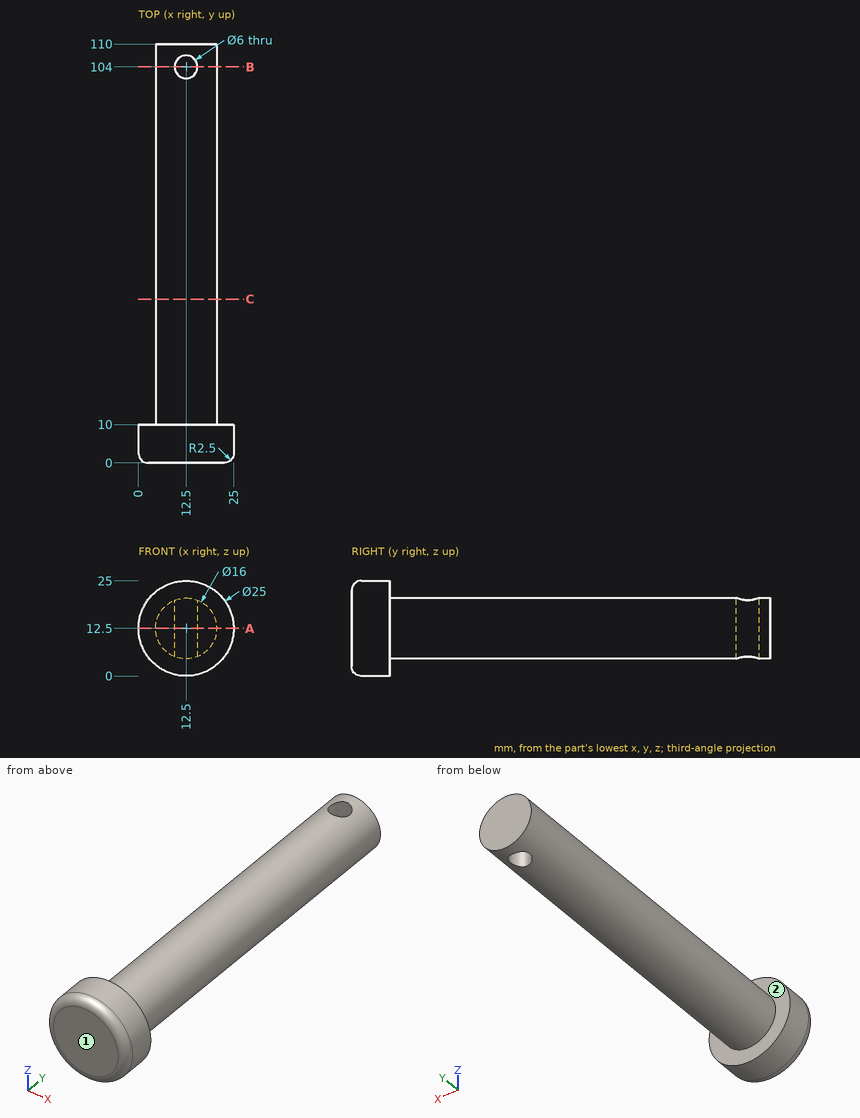
The drawing under review shows one solid part. Ordinate dimensions are in mm from its lowest x, y, z. A direction names the side the tool comes from. Give positions to 0.01 mm unless a question says otherwise; leave off trailing zeros. Write each loop counter-clockwise with the first axis right and the second up, starting at its lowest first coordinate (ties: lowest second). Pieces come first, ordered by that corner, then holes. Notation, with made-up numbers: M -3.5,45.25 L 26.5,45.25 A17 cw 26.5,64.25 Z; hole C 66,66.5 d1. An arc over 180 degrees is marked long. Write each question's results on one line, items separated by ' | '. Start each with the question number.
1. We need section A-A (z = 12.5). Write out the cut boundary in (x, y).
2. For probe 1 along Y at (x, z) = (12.5, 16); probe 2 along X at (y, z) = (104, 16); probe 3 along Y at (x, z) = (3, 16.25), list the stretches that pass through material, from the lowest coordinate up. Write a range as [from, to].
3. We need section B-B (y = 104). Write out the cut boundary in (x, z), and give its area (3 significant figures).
4. Insertion check: pin 1 Ø2 at (y, z) = (47.5, 20.5) entering from -X; pin 2 Ø12 at (x, y) = (20.5, 93.5) entering from +Z; pin 3 Ø12 at (y, z) = (77.5, 13) entering from -X; pin 4 Ø1.5 at (x, y) = (22, 18.5) entering from -Z. Each pin has a flat end and moves straight along its axis. Give the tip position at first contact, or say it passes through.
5. We need section C-C (y = 43). Write out the cut boundary in (x, z), and give its area (3 significant figures).
6. For the marked faces 1 and 2, list the 3-axis set-ups (+Z, -Z, +X, -X, +Y, -Y) from which the entire face can be reached by the end or side of a thin tool; tool diameter is ignored.
Results found:
1) outline: M 0,2.5 A2.5 ccw 2.5,0 L 22.5,0 A2.5 ccw 25,2.5 L 25,10 L 20.5,10 L 20.5,110 L 4.5,110 L 4.5,10 L 0,10 Z; hole C 12.5,104 d6
2) probe 1: y = [0, 101], [107, 110] | probe 2: x = [5.31, 9.5], [15.5, 19.69] | probe 3: y = [0.01, 10]
3) outline: M 9.5,5.08 L 9.5,19.92 A8 ccw Z; M 15.5,5.08 A8 ccw 15.5,19.92 Z | area: 107 mm^2
4) pin 1: stops at x = 8.63 | pin 2: stops at z = 20.25 | pin 3: stops at x = 4.5 | pin 4: passes through
5) outline: C 12.5,12.5 d16 | area: 201 mm^2
6) face 1: +Z, -Z, +X, -X, -Y | face 2: +Y
